Geometry: final body of the model. Coordinates: model frame, mm. A direction names the side the tool comes from. Give positions to 0.01 mm unless a question says otherwise; leave off trailing zeros. Order: outer loops, then holes, each group sorted by start corner. A loop starts at its lowest first (then second) coordinate and runs counter-clockwise, first axis right, second up. Notation, with made-up numbers: (67.5, 79.25) -> (74.5, 79.25) arc R9 cw to (74.5, 88.25) -> close; hole circle Ø7 at (38, 1). An arc over 180 degrees is marked (long way). One line per question, with ' | ' between items. Start each with the question number.
(1) Ray query, L1, parallel to X at y = -234, z = 666.5; L2, parallel to Z at x = 154, y = -205; L3, parallel to Y at x = 11, z = 574.5. Return the intervals inside material, ascending.
(2) Set-up query: faces 4 (the face through (228.6, -157, 382)), 5 (the face through (-214.312, -147, 382)). Return all of +Z, -Z, +X, -X, +Y, -Y with unobstructed straight access to the full face (end or side cutting, diameter ignored); none if empty.
(3) First-contact query: pin 1 Ø8 at (x, y) = (96.84, -39.69) entering from +Z; pin 2 Ø4 at (x, y) = (157.16, -39.69) entering from +Z; pin 3 Ø4 at (y, z) = (-263.525, 238.125) entering from -X; pin 4 Ø2.5 at (y, z) = (6, 491) entering from +X. Flat tips, straight axial feed; report the tip coordinate or a pass-through.
(4) Section A-A (y = -179). Return loops of the section in (x, z), then the cut area to 3 significant figures.
(5) Section C-C (x = -16). Return loops of the section in (y, z).
(6) Mould query, pull axis Z, two halves, no side actions, for faces 1 (the face through (-3, -148, 774.7)), 2 (the face through (-3, -147, 38.1)), 3 (the face through (220, 0, 389)). Classes: +Z half, -Z half, draft (parallel to the pull), parting line (faces both ways), or undercut.
```python
from build123d import *

# Parameters (mm, degrees)
F0_W      = 457.2
F0_H      = 774.7
F1_DEPTH  = 317.5
F2_W      = 381
F2_H      = 698.5
F3_W      = 428.625
F3_H      = 698.5
F4_DEPTH  = 298.45
F5_START  = 19.05
F5_DEPTH  = 279.4
F7_DEPTH  = 774.7
F9_D      = 4.9149
F9_DEPTH  = 38.1
F9_TIP    = 1.4765849282
F10_R     = 2.413
F11_DEPTH = 25.4


# Not quite as in the source:
# - a feature names something its author has since deleted; it is built from what else it names


with BuildPart() as f1:
    # F0 (on Front) → F1 (new body)
    with BuildSketch(Plane.XZ):
        with Locations((0, 387.35)):
            Rectangle(F0_W, F0_H)
    extrude(amount=F1_DEPTH)

    # F2 (on Front) + F3 (on Front) → F4 (cut)
    with BuildSketch(Plane.XZ):
        with Locations((0, 387.35)):
            Rectangle(F2_W, F2_H)
    with BuildSketch(Plane.XZ):
        with Locations((0, 387.35)):
            Rectangle(F3_W, F3_H)
    extrude(amount=F4_DEPTH, mode=Mode.SUBTRACT)

    # F3 (on Front) → F5 (cut)
    with BuildSketch(Plane.XZ.offset(F5_START)):
        with Locations((0, 387.35)):
            Rectangle(F3_W, F3_H)
    extrude(amount=F5_DEPTH, mode=Mode.SUBTRACT)

    # F6 (on Top) → F7 (join, through all)
    with BuildSketch(Plane.XY):
        with BuildLine():
            Line((-204.7875, 0), (-204.7875, 8.2098719395))
            ThreePointArc((-204.7875, 8.2098719395), (-206.375, 17.4625), (-207.9625, 8.2098719395))
            Line((-207.9625, 8.2098719395), (-207.9625, 0))
            Line((-207.9625, 0), (-204.7875, 0))
        make_face()
    extrude(amount=F7_DEPTH)

    # F9
    with Locations(Plane.XY.offset(774.7)):
        with Locations((96.8375, -153.9875), (157.1625, -39.6875), (157.1625, -153.9875), (96.8375, -268.2875), (96.8375, -39.6875), (157.1625, -268.2875)):
            Hole(F9_D / 2, depth=F9_DEPTH)
            with Locations((0, 0, -(F9_DEPTH + F9_TIP / 2))):  # 118° drill point
                Cone(0, F9_D / 2, F9_TIP, mode=Mode.SUBTRACT)

    # F10 (on face) → F11 (cut)
    with BuildSketch(Plane(origin=(-228.6, 0, 0), x_dir=(0, -1, 0), z_dir=(-1, 0, 0))):
        with Locations((34.925, 695.325)):
            Circle(F10_R)
        with Locations((34.925, 527.05)):
            Circle(F10_R)
        with Locations((34.925, 466.725)):
            Circle(F10_R)
        with Locations((34.925, 298.45)):
            Circle(F10_R)
        with Locations((34.925, 238.125)):
            Circle(F10_R)
        with Locations((34.925, 69.85)):
            Circle(F10_R)
        with Locations((263.525, 69.85)):
            Circle(F10_R)
        with Locations((263.525, 238.125)):
            Circle(F10_R)
        with Locations((263.525, 298.45)):
            Circle(F10_R)
        with Locations((263.525, 466.725)):
            Circle(F10_R)
        with Locations((263.525, 527.05)):
            Circle(F10_R)
        with Locations((263.525, 695.325)):
            Circle(F10_R)
    extrude(amount=-F11_DEPTH, mode=Mode.SUBTRACT)


solid = f1.part
```
Response:
1) L1: x = -228.6 to -214.31, 214.31 to 228.6 | L2: z = 0 to 38.1, 736.6 to 774.7 | L3: y = -317.5 to -298.45
2) face 4: +Z, -Z, +X, +Y, -Y | face 5: +Y
3) pin 1: stops at z = 774.7 | pin 2: stops at z = 38.1 | pin 3: stops at x = 214.31 | pin 4: stops at x = -204.79
4) outline: (-228.6, 0) -> (228.6, 0) -> (228.6, 774.7) -> (-228.6, 774.7) -> close; hole (-214.31, 38.1) -> (214.31, 38.1) -> (214.31, 736.6) -> (-214.31, 736.6) -> close | area: 54,800 mm^2
5) outline: (-317.5, 0) -> (0, 0) -> (0, 38.1) -> (-298.45, 38.1) -> (-298.45, 736.6) -> (0, 736.6) -> (0, 774.7) -> (-317.5, 774.7) -> close
6) face 1: +Z half | face 2: undercut | face 3: draft
